Work out the finished part from the listing and answer in its coordinate system (mm). A direction names the side the tool comes from. Coordinates: 2 decimals unless noted, no trailing zeros. Order: outer loops, then holes, each group sorted by start corner. A loop starts at its lowest first (then second) coordinate and runs counter-clockwise, first axis right, second up. Notation, with made-up numbers: M 24.25,49 L 78.25,49 A24 ccw 78.25,86 Z; hole C 25,-10 d10. An arc over 180 degrees is marked long. Answer in a Markdown table with one row per item. Add a question column.
Item 1: Which of the six approach directions +Z, -Z, +X, -X, +Y, -Y give full straight-line access (tool end or side, diameter ignored) to faces 4 (the face through (-6.604, 0, -1)), 5 (the face through (0, 1, 2.54)), 6 (the face through (13, 0, -2.54))?
Item 2: The part is cut by section A-A (z = 6). Write down the section's boundary in (x, y) (3 decimals).
Item 3: Flat-ended cylindrical pins translate along their axes: pin 1 Ø3 at (y, z) = (-15.5, 7.5) entering from -X; pin 2 Ø4 at (x, z) = (-17.5, 2) entering from +Y; pin 3 Ø1 at (x, z) = (2.5, 9) entering from +Y. Find the tip coordinate at first contact, or state that the pin passes through.
Item 4: Consider line 1 (Z direction, x = -23, y = 2); line 2 (Y direction, x = 6, z = 5.5); line 3 (X direction, y = 7, z = -0.5). Determine where each line is inside the solid, lowest interval first. Write a range as from..to.
Item 5: The mould has two halves that part along X. Classify faces 1 (the face through (7.4, -22.5, 10.16)), 2 (the face through (-23.49, 0.42, -1.25)), 3 (the face through (6.604, 0, -1)): released by +X, released by -X, zero draft, split by the parting line, or undercut.
Item 6: The part is cut by section D-D (x = -17). Write down the section's boundary in (y, z).
Item 7: The part is cut by section C-C (y = 1.5). Write down the section's boundary in (x, z), then the cut area to 3 significant figures.
Item 8: The part is cut by section B-B (x = 4). Write down the section's boundary in (y, z), then the cut area to 3 significant figures.
from build123d import *

# Parameters (mm, degrees)
F0_R     = 25.4
F1_DEPTH = 10.16
F2_DEPTH = 2.54
F3_DEPTH = 2.54


with BuildPart() as f1:
    # F0 (on Top) → F1 (new body)
    with BuildSketch(Plane.XY):
        Circle(F0_R)
        with BuildLine():
            ThreePointArc((0, -23.495), (-3.3357925983, -23.256988471), (-6.604, -22.5477761431))
            ThreePointArc((-6.604, -22.5477761431), (-23.495, 0), (-6.604, 22.5477761431))
            Line((-6.604, 22.5477761431), (-6.604, 23.495))
            Line((-6.604, 23.495), (0, 23.495))
            Line((0, 23.495), (6.604, 23.495))
            Line((6.604, 23.495), (6.604, 22.5477761431))
            ThreePointArc((6.604, 22.5477761431), (18.8039358247, 14.086412691), (23.495, 0))
            ThreePointArc((23.495, 0), (18.8039358247, -14.086412691), (6.604, -22.5477761431))
            ThreePointArc((6.604, -22.5477761431), (3.3357925983, -23.256988471), (0, -23.495))
        make_face(mode=Mode.SUBTRACT)
        with BuildLine():
            Line((-6.604, 23.495), (-6.604, 22.5477761431))
            ThreePointArc((-6.604, 22.5477761431), (-3.3357925983, 23.256988471), (0, 23.495))
            Line((0, 23.495), (-6.604, 23.495))
        make_face()
        with BuildLine():
            Line((6.604, 23.495), (0, 23.495))
            ThreePointArc((0, 23.495), (3.3357925983, 23.256988471), (6.604, 22.5477761431))
            Line((6.604, 22.5477761431), (6.604, 23.495))
        make_face()
    extrude(amount=F1_DEPTH)

    # F0 (on Top) → F2 (join)
    with BuildSketch(Plane.XY):
        with BuildLine():
            ThreePointArc((-6.604, 22.5477761431), (-23.495, 0), (-6.604, -22.5477761431))
            Line((-6.604, -22.5477761431), (-6.604, 22.5477761431))
        make_face()
        with BuildLine():
            Line((-6.604, 22.5477761431), (-6.604, -22.5477761431))
            Line((-6.604, -22.5477761431), (0, -22.5477761431))
            Line((0, -22.5477761431), (0, 23.495))
            ThreePointArc((0, 23.495), (-3.3357925983, 23.256988471), (-6.604, 22.5477761431))
        make_face()
        with BuildLine():
            Line((0, 23.495), (0, -22.5477761431))
            Line((0, -22.5477761431), (6.604, -22.5477761431))
            Line((6.604, -22.5477761431), (6.604, 22.5477761431))
            ThreePointArc((6.604, 22.5477761431), (3.3357925983, 23.256988471), (0, 23.495))
        make_face()
        with BuildLine():
            Line((6.604, 22.5477761431), (6.604, -22.5477761431))
            ThreePointArc((6.604, -22.5477761431), (18.8039358247, -14.086412691), (23.495, 0))
            ThreePointArc((23.495, 0), (18.8039358247, 14.086412691), (6.604, 22.5477761431))
        make_face()
    extrude(amount=F2_DEPTH)

    # F0 (on Top) → F3 (join)
    with BuildSketch(Plane.XY):
        with BuildLine():
            ThreePointArc((-6.604, 22.5477761431), (-23.495, 0), (-6.604, -22.5477761431))
            Line((-6.604, -22.5477761431), (-6.604, 22.5477761431))
        make_face()
        with BuildLine():
            Line((6.604, 22.5477761431), (6.604, -22.5477761431))
            ThreePointArc((6.604, -22.5477761431), (18.8039358247, -14.086412691), (23.495, 0))
            ThreePointArc((23.495, 0), (18.8039358247, 14.086412691), (6.604, 22.5477761431))
        make_face()
    extrude(amount=-F3_DEPTH)


solid = f1.part
Reply:
| question | item | result |
|---|---|---|
| 1 | face 4 | -Z, +Y, -Y |
| 1 | face 5 | +Z |
| 1 | face 6 | -Z, +X, -X, +Y, -Y |
| 2 | outline | C 0,0 d50.8; hole C 0,0 d46.99 |
| 3 | pin 1 | stops at x = -21.19 |
| 3 | pin 2 | stops at y = 20.12 |
| 3 | pin 3 | stops at y = 25.32 |
| 4 | line 1 | z = -2.54..2.54 |
| 4 | line 2 | y = -24.68..-22.72, 22.72..24.68 |
| 4 | line 3 | x = -22.43..-6.6, 6.6..22.43 |
| 5 | face 1 | zero draft |
| 5 | face 2 | released by -X |
| 5 | face 3 | undercut |
| 6 | outline | M -18.87,0 L -16.22,0 L -16.22,-2.54 L 16.22,-2.54 L 16.22,0 L 18.87,0 L 18.87,10.16 L 16.22,10.16 L 16.22,2.54 L -16.22,2.54 L -16.22,10.16 L -18.87,10.16 Z |
| 7 | outline | M -25.36,0 L -23.45,0 L -23.45,-2.54 L -6.6,-2.54 L -6.6,0 L 6.6,0 L 6.6,-2.54 L 23.45,-2.54 L 23.45,0 L 25.36,0 L 25.36,10.16 L 23.45,10.16 L 23.45,2.54 L -23.45,2.54 L -23.45,10.16 L -25.36,10.16 Z |
| 7 | area | 243 mm2 |
| 8 | outline | M -25.08,0 L -23.15,0 L -23.15,10.16 L -25.08,10.16 Z; M -22.55,0 L 25.08,0 L 25.08,10.16 L 23.15,10.16 L 23.15,2.54 L -22.55,2.54 Z |
| 8 | area | 155 mm2 |
